Part model, mm, in its own coordinate system. Face numbers are marked on the shaded views. A direction names the side the tool comes from. Round coordinates to 2 decimals unless told otherwise and drop trailing zeros. Write each loop counter-clockwise with the first axis right and the second up, starting at its lowest first coordinate (ties: lowest second). Pieces come first, ordered by that corner, then holes.
1) Saw through at D-D on z = -2.5. Write the cut outline in (x, y).
2) Drill centre lines: L1, parallel to X at y = 0.1, z = 24.5; L2, parallel to Z at x = 1.1, y = -0.1; L3, parallel to Z at x = 0.55, y = -1.8. Where is each one in solid material? Low to high.
3) Saw through at B-B on y = 0. Write the cut outline in (x, z).
4) Saw through at C-C on x = -1.05. Write the cut outline in (y, z).
5) Flat gauge pin, fed straight in: pin 1 (2 mm diameter, centred on x = -2, z = 8, fed in from -Y). Where does the tip first touch, or does it go through?
6) Which spindle directions (+Z, -Z, +X, -X, +Y, -Y) get a long thin tool onto all of the face, cutting with end or side? Do the marked faces 1 and 2. Say none if no direction does.
7) Saw through at A-A on z = 18. Write the cut outline in (x, y).
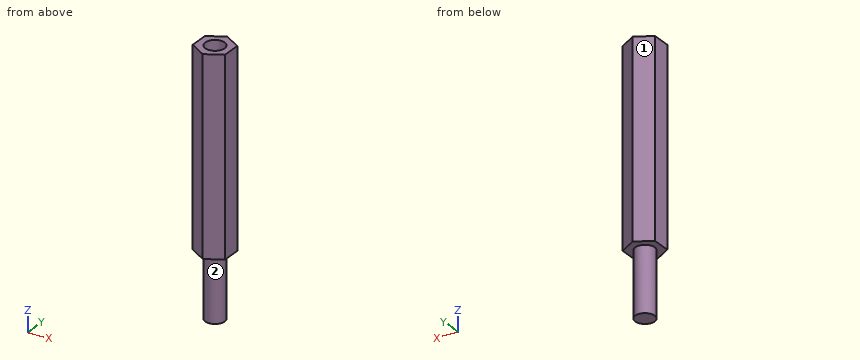
```python
from build123d import *

# Parameters (mm, degrees)
ESQUISSE1_R             = 1.5
BOSS_EXTRU_2_DEPTH      = 30
ESQUISSE3_R             = 1.5
BOSS_EXTRU_3_DEPTH      = 10
BOSS_EXTRU_3_DEPTH_BACK = 20


with BuildPart() as part:
    # Esquisse1 → Boss.-Extru.2 (new body)
    with BuildSketch(Plane.XY):
        Polygon((0, -2.886751346), (2.5, -1.443375673), (2.5, 1.443375673), (0, 2.886751346), (-2.5, 1.443375673), (-2.5, -1.443375673), align=None)
        Circle(ESQUISSE1_R, mode=Mode.SUBTRACT)
    extrude(amount=BOSS_EXTRU_2_DEPTH)

    # Esquisse3 → Boss.-Extru.3 (add, two sides)
    with BuildSketch(Plane(origin=(0, 0, 0), x_dir=(-1, 0, 0), z_dir=(0, 0, -1))) as boss_extru_3_sk:
        Circle(ESQUISSE3_R)
    extrude(amount=BOSS_EXTRU_3_DEPTH)
    extrude(boss_extru_3_sk.sketch, amount=-BOSS_EXTRU_3_DEPTH_BACK)


solid = part.part
```
Completed:
1. outline: circle Ø3 at (0, 0)
2. L1: x = -2.5 to -1.5, 1.5 to 2.5
2. L2: z = -10 to 20
2. L3: z = 0 to 30
3. outline: (-2.5, 0) - (-1.5, 0) - (-1.5, -10) - (1.5, -10) - (1.5, 0) - (2.5, 0) - (2.5, 30) - (1.5, 30) - (1.5, 20) - (-1.5, 20) - (-1.5, 30) - (-2.5, 30) - close
4. outline: (-2.28, 0) - (-1.07, 0) - (-1.07, -10) - (1.07, -10) - (1.07, 0) - (2.28, 0) - (2.28, 30) - (1.07, 30) - (1.07, 20) - (-1.07, 20) - (-1.07, 30) - (-2.28, 30) - close
5. pin 1: stops at y = -2.31
6. face 1: +Z, -Z, -X, +Y
6. face 2: -Z
7. outline: (-2.5, -1.44) - (0, -2.89) - (2.5, -1.44) - (2.5, 1.44) - (0, 2.89) - (-2.5, 1.44) - close
